The model under review builds one solid part; all positions refer to its coordinate system, in mm. Face numbers are marked on the shaded views. Give positions to 0.01 mm unless a question says otherwise; leave off trailing zeros. Loops run counter-clockwise (first coordinate to the right, second up) from the corner with the lowest first, then second, coordinate; pieces in that order, holes last. Notation, with made-up numbers: M -32,-40 L -27,-40 A23 cw -27,-5 Z; hole C 35.25,-5.5 d5. An arc over 180 degrees is marked long. Return JSON: item names as keys, results as strings.
```python
from build123d import *

# Parameters (mm, degrees)
SKETCH3_W             = 32
SKETCH3_H             = 50
BOSS_EXTRUDE1_DEPTH   = 5
CUT_W                 = 20
CUT_H                 = 6.55
CUT_EXTRUDE1_DEPTH    = 10
SKETCH4_W             = 25.5
SKETCH4_H             = 50
BOSS_EXTRUDE2_DEPTH   = 5
SKETCH5_W             = 5
SKETCH5_H             = 50
BOSS_EXTRUDE3_DEPTH   = 51
BOSS_EXTRUDE4_REACH   = 80
SKETCH6_W             = 5
SKETCH6_H             = 50
BOSS_EXTRUDE5_DEPTH   = 5
FILLET1_R             = 10
BOSS_EXTRUDE6_DEPTH   = 5
SKETCH9_W             = 5
SKETCH9_H             = 15
BOSS_EXTRUDE7_DEPTH   = 2.5
BOSS_EXTRUDE8_DEPTH   = 5
SKETCH11_R            = 1
CUT_EXTRUDE2_DEPTH    = 5
FILLET4_R             = 5
FILLET5_R             = 5
CHAMFER1_SIZE         = 5
CHAMFER1_SIZE2        = 8.660254038
CHAMFER1_PART_2_SIZE  = 5
CHAMFER1_PART_2_SIZE2 = 8.660254038
FILLET6_R             = 5
CHAMFER2_SIZE         = 5
CHAMFER2_SIZE2        = 8.660254038
CHAMFER2_PART_2_SIZE  = 5
CHAMFER2_PART_2_SIZE2 = 8.660254038
SKETCH12_R            = 2.5
CUT_EXTRUDE3_DEPTH    = 57


with BuildPart() as part:
    # Sketch3 → Boss-Extrude1 (new body)
    with BuildSketch(Plane(origin=(0, 0, -16), x_dir=(-1, 0, 0), z_dir=(0, 0, -1))):
        with Locations((0, -13.5)):
            Rectangle(SKETCH3_W, SKETCH3_H)
    extrude(amount=BOSS_EXTRUDE1_DEPTH)

    # Cut → Cut-Extrude1 (cut)
    with BuildSketch(Plane(origin=(0, 0, -16), x_dir=(-1, 0, 0), z_dir=(0, 0, -1))):
        with BuildLine():
            Line((9.2, -32.5), (4.8, -32.5))
            ThreePointArc((4.8, -32.5), (4.234314575, -32.265685425), (4, -31.7))
            Line((4, -31.7), (4, -26.1))
            ThreePointArc((4, -26.1), (4.234314575, -25.534314575), (4.8, -25.3))
            Line((4.8, -25.3), (9.2, -25.3))
            ThreePointArc((9.2, -25.3), (9.765685425, -25.534314575), (10, -26.1))
            Line((10, -26.1), (10, -31.7))
            ThreePointArc((10, -31.7), (9.765685425, -32.265685425), (9.2, -32.5))
        make_face()
        with BuildLine():
            Line((-10, -31.7), (-10, -26.1))
            ThreePointArc((-10, -26.1), (-9.765685425, -25.534314575), (-9.2, -25.3))
            Line((-9.2, -25.3), (-4.8, -25.3))
            ThreePointArc((-4.8, -25.3), (-4.234314575, -25.534314575), (-4, -26.1))
            Line((-4, -26.1), (-4, -31.7))
            ThreePointArc((-4, -31.7), (-4.234314575, -32.265685425), (-4.8, -32.5))
            Line((-4.8, -32.5), (-9.2, -32.5))
            ThreePointArc((-9.2, -32.5), (-9.765685425, -32.265685425), (-10, -31.7))
        make_face()
        with Locations((0, -15.375)):
            Rectangle(CUT_W, CUT_H)
        with BuildLine():
            ThreePointArc((-5.5, 0), (0, -5.5), (5.5, 0))
            ThreePointArc((5.5, 0), (0, 5.5), (-5.5, 0))
        make_face()
        with BuildLine():
            ThreePointArc((13.5, -7.6), (14.6, -6.500000002), (13.500000003, -5.4))
            ThreePointArc((13.500000003, -5.4), (12.4, -6.499999998), (13.5, -7.6))
        make_face()
        with BuildLine():
            ThreePointArc((13.5, -31.6), (14.6, -30.500000002), (13.500000003, -29.4))
            ThreePointArc((13.500000003, -29.4), (12.4, -30.499999998), (13.5, -31.6))
        make_face()
        with BuildLine():
            ThreePointArc((-13.5, -31.6), (-12.4, -30.499999998), (-13.500000003, -29.4))
            ThreePointArc((-13.500000003, -29.4), (-14.6, -30.500000002), (-13.5, -31.6))
        make_face()
        with BuildLine():
            ThreePointArc((-13.5, -7.6), (-12.4, -6.499999998), (-13.500000003, -5.4))
            ThreePointArc((-13.500000003, -5.4), (-14.6, -6.500000002), (-13.5, -7.6))
        make_face()
    extrude(amount=CUT_EXTRUDE1_DEPTH, mode=Mode.SUBTRACT)

    # Sketch4 → Boss-Extrude2 (add)
    with BuildSketch(Plane(origin=(0, 0, -21), x_dir=(-1, 0, 0), z_dir=(0, 0, -1))):
        with Locations((-28.75, -13.5)):
            Rectangle(SKETCH4_W, SKETCH4_H)
        with Locations((28.75, -13.5)):
            Rectangle(SKETCH4_W, SKETCH4_H)
    extrude(amount=-BOSS_EXTRUDE2_DEPTH)

    # Sketch5 → Boss-Extrude3 (add)
    with BuildSketch(Plane.XY.offset(-16)):
        with Locations((-39, -13.5)):
            Rectangle(SKETCH5_W, SKETCH5_H)
        with Locations((39, -13.5)):
            Rectangle(SKETCH5_W, SKETCH5_H)
    extrude(amount=BOSS_EXTRUDE3_DEPTH)

    # Sketch6 → Boss-Extrude4 (add, up to next)
    with BuildSketch(Plane.ZY.offset(-36.5), mode=Mode.PRIVATE) as boss_extrude4_sk1:
        with Locations((32.5, -13.5)):
            Rectangle(SKETCH6_W, SKETCH6_H)
    boss_extrude4_tool1 = extrude(boss_extrude4_sk1.sketch, amount=BOSS_EXTRUDE4_REACH, mode=Mode.PRIVATE) - part.part
    add(boss_extrude4_tool1.solids().sort_by_distance((36.5, -13.5, 32.5))[0])

    # Sketch7 → Boss-Extrude5 (add)
    with BuildSketch(Plane(origin=(0, 0, -21), x_dir=(-1, 0, 0), z_dir=(0, 0, -1))):
        with BuildLine():
            Line((-11.859707003, 40.449348023), (-21.5, 11.5))
            Line((-21.5, 11.5), (21.5, 11.5))
            Line((21.5, 11.5), (11.859707003, 40.449348023))
            ThreePointArc((11.859707003, 40.449348023), (0, 49), (-11.859707003, 40.449348023))
        make_face()
    extrude(amount=-BOSS_EXTRUDE5_DEPTH)

    # Fillet1
    fillet1_edges = [part.edges().sort_by_distance(p)[0] for p in [
        (-21.5, 11.5, -18.5),
        (21.5, 11.5, -18.5),
    ]]
    fillet(fillet1_edges, radius=FILLET1_R)

    # Sketch8 → Boss-Extrude6 (add)
    with BuildSketch(Plane.XY.offset(35)):
        with BuildLine():
            Line((11.859707003, 40.449348023), (19.222068481, 18.340521582))
            ThreePointArc((19.222068481, 18.340521582), (22.86153451, 13.388440835), (28.709834084, 11.5))
            Line((28.709834084, 11.5), (-28.709834084, 11.5))
            ThreePointArc((-28.709834084, 11.5), (-22.86153451, 13.388440835), (-19.222068481, 18.340521582))
            Line((-19.222068481, 18.340521582), (-11.859707003, 40.449348023))
            ThreePointArc((-11.859707003, 40.449348023), (0, 49), (11.859707003, 40.449348023))
        make_face()
    extrude(amount=-BOSS_EXTRUDE6_DEPTH)

    # Sketch9 → Boss-Extrude7 (add, symmetric)
    with BuildSketch(Plane(origin=(16.5, 0, 0), x_dir=(0, 0, -1), z_dir=(1, 0, 0))):
        with Locations((-32.5, -46)):
            Rectangle(SKETCH9_W, SKETCH9_H)
        with Locations((18.5, -46)):
            Rectangle(SKETCH9_W, SKETCH9_H)
    extrude(amount=BOSS_EXTRUDE7_DEPTH, both=True)

    # Sketch10 → Boss-Extrude8 (add)
    with BuildSketch(Plane(origin=(19, 0, 0), x_dir=(0, 0, -1), z_dir=(1, 0, 0))):
        with BuildLine():
            Line((-30, -53.5), (-18, -53.5))
            ThreePointArc((-18, -53.5), (-7, -64.5), (4, -53.5))
            Line((4, -53.5), (16, -53.5))
            Line((16, -53.5), (16, -43.5))
            Line((16, -43.5), (-2.417424305, -43.5))
            ThreePointArc((-2.417424305, -43.5), (-7, -42.5), (-11.582575695, -43.5))
            Line((-11.582575695, -43.5), (-30, -43.5))
            Line((-30, -43.5), (-30, -53.5))
        make_face()
    extrude(amount=-BOSS_EXTRUDE8_DEPTH)

    # Sketch11 → Cut-Extrude2 (cut)
    with BuildSketch(Plane(origin=(19, 0, 0), x_dir=(0, 0, -1), z_dir=(1, 0, 0))):
        with Locations((-15, -53.5)):
            Circle(SKETCH11_R)
        with Locations((-7, -45.5)):
            Circle(SKETCH11_R)
        with Locations((1, -53.5)):
            Circle(SKETCH11_R)
        with Locations((-7, -61.5)):
            Circle(SKETCH11_R)
    extrude(amount=-CUT_EXTRUDE2_DEPTH, mode=Mode.SUBTRACT)

    # Fillet4
    fillet4_edges = [part.edges().sort_by_distance(p)[0] for p in [
        (41.5, -13.5, -21),
        (-41.5, -13.5, -21),
        (-41.5, -13.5, 35),
        (41.5, -13.5, 35),
    ]]
    fillet(fillet4_edges, radius=FILLET4_R)

    # Fillet5
    fillet5_edges = [part.edges().sort_by_distance(p)[0] for p in [
        (16.5, -53.5, 35),
        (16.5, -53.5, -21),
    ]]
    fillet(fillet5_edges, radius=FILLET5_R)

    # Chamfer1
    chamfer1_edges = [part.edges().sort_by_distance(p)[0] for p in [
        (16.5, -43.5, -16),
    ]]
    chamfer1_side = [part.faces().sort_by_distance(p)[0] for p in [
        (-22.17239609, 12.432609658, -16),
    ]]
    chamfer(chamfer1_edges, length=CHAMFER1_SIZE, length2=CHAMFER1_SIZE2, reference=chamfer1_side[0])

    # Chamfer1 part 2
    chamfer1_part_2_edges = [part.edges().sort_by_distance(p)[0] for p in [
        (16.5, -43.5, 30),
    ]]
    chamfer1_part_2_side = [part.faces().sort_by_distance(p)[0] for p in [
        (0.085787805, -4.114556323, 30),
    ]]
    chamfer(chamfer1_part_2_edges, length=CHAMFER1_PART_2_SIZE, length2=CHAMFER1_PART_2_SIZE2, reference=chamfer1_part_2_side[0])

    # Fillet6
    fillet6_edges = [part.edges().sort_by_distance(p)[0] for p in [
        (16.5, -38.5, -16),
        (16.5, -38.5, 30),
    ]]
    fillet(fillet6_edges, radius=FILLET6_R)

    # Chamfer2
    chamfer2_edges = [part.edges().sort_by_distance(p)[0] for p in [
        (14, -38.5, 32.5),
        (14, -38.5, -18.5),
    ]]
    chamfer2_side = [part.faces().sort_by_distance(p)[0] for p in [
        (14, -49.7166158, 7),
    ]]
    chamfer(chamfer2_edges, length=CHAMFER2_SIZE, length2=CHAMFER2_SIZE2, reference=chamfer2_side[0])

    # Chamfer2 part 2
    chamfer2_part_2_edges = [part.edges().sort_by_distance(p)[0] for p in [
        (19, -38.5, 32.5),
        (19, -38.5, -18.5),
    ]]
    chamfer2_part_2_side = [part.faces().sort_by_distance(p)[0] for p in [
        (19, -49.7166158, 7),
    ]]
    chamfer(chamfer2_part_2_edges, length=CHAMFER2_PART_2_SIZE, length2=CHAMFER2_PART_2_SIZE2, reference=chamfer2_part_2_side[0])

    # Sketch12 → Cut-Extrude3 (cut, through all)
    with BuildSketch(Plane.XY.offset(35)):
        with Locations((0, 36.5)):
            Circle(SKETCH12_R)
    extrude(amount=-CUT_EXTRUDE3_DEPTH, mode=Mode.SUBTRACT)


solid = part.part
```
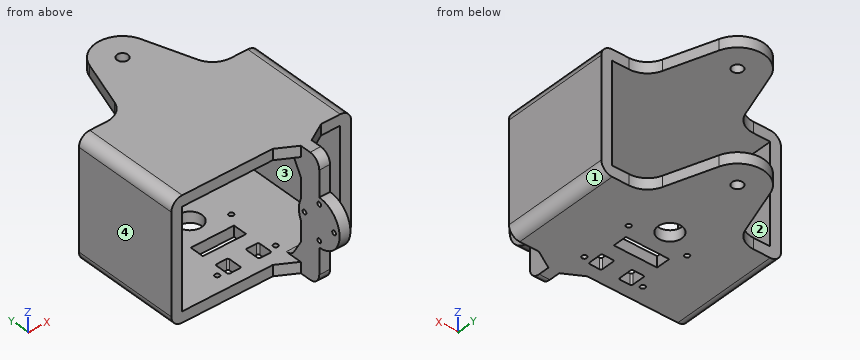
1) Consider section C-C on x = 32. Write out the cut boundary in (y, z), then the cut area to 3 significant figures.
From the geometry:
{"outline": "M -38.5,-21 L 11.5,-21 L 11.5,-16 L -38.5,-16 Z; M -38.5,30 L 11.5,30 L 11.5,35 L -38.5,35 Z", "area": "500 mm²"}
2) Wall thickness on L1, parallel to Y at x = 0, z = -17; L2, parallel to Z at x = 25, y = -37.5; L3, parallel to X at y = 6.5, z = -6: over which ranges is each line inside the solid? List them lowest first. Write a range as from..to.
From the geometry:
{"L1": "-38.5..-18.65, -12.1..-5.5, 5.5..34, 39..49", "L2": "-21..-16, 30..35", "L3": "-41.5..-36.5, 36.5..41.5"}
3) Consider section D-D on y = 0. Write out the cut boundary in (x, z).
From the geometry:
{"outline": "M -41.5,-16 A5 ccw -36.5,-21 L -5.5,-21 L -5.5,-16 L -36.5,-16 L -36.5,30 L 36.5,30 L 36.5,-16 L 5.5,-16 L 5.5,-21 L 36.5,-21 A5 ccw 41.5,-16 L 41.5,30 A5 ccw 36.5,35 L -36.5,35 A5 ccw -41.5,30 Z"}
4) Consider section B-B on y = 27.5. Write out the cut boundary in (x, z), then the cut area to 3 significant figures.
From the geometry:
{"outline": "M -16.17,-21 L 16.17,-21 L 16.17,-16 L -16.17,-16 Z; M -16.17,30 L 16.17,30 L 16.17,35 L -16.17,35 Z", "area": "323 mm²"}
5) Insertion check: pin 1 (2.5 mm diameter, centred on x = 16.5, z = -9.5, fed in from -Y); pin 2 (2.5 mm diameter, centred on x = 16, z = 0, fed in from +Y); pin 3 (10 mm diameter, centred on x = 0, y = 0, fed in from -Z). Each pin has a flat end and moves straight along its axis. Give the tip position at first contact, or say it passes through.
From the geometry:
{"pin 1": "y = -53.5", "pin 2": "y = -43.5", "pin 3": "z = 30"}
6) The part is to be moulded in two halves that separate along Z. For the marked faces 1, 2, 3 and 4, say which applies: released by +Z, released by -Z, zero draft, split by the parting line, or undercut.
From the geometry:
{"face 1": "released by -Z", "face 2": "undercut", "face 3": "undercut", "face 4": "zero draft"}
7) Consider section A-A on x = 0. Write out the cut boundary in (y, z).
From the geometry:
{"outline": "M -38.5,-21 L -18.65,-21 L -18.65,-16 L -38.5,-16 Z; M -38.5,30 L 34,30 L 34,35 L -38.5,35 Z; M -12.1,-21 L -5.5,-21 L -5.5,-16 L -12.1,-16 Z; M 5.5,-21 L 34,-21 L 34,-16 L 5.5,-16 Z; M 39,-21 L 49,-21 L 49,-16 L 39,-16 Z; M 39,30 L 49,30 L 49,35 L 39,35 Z"}
